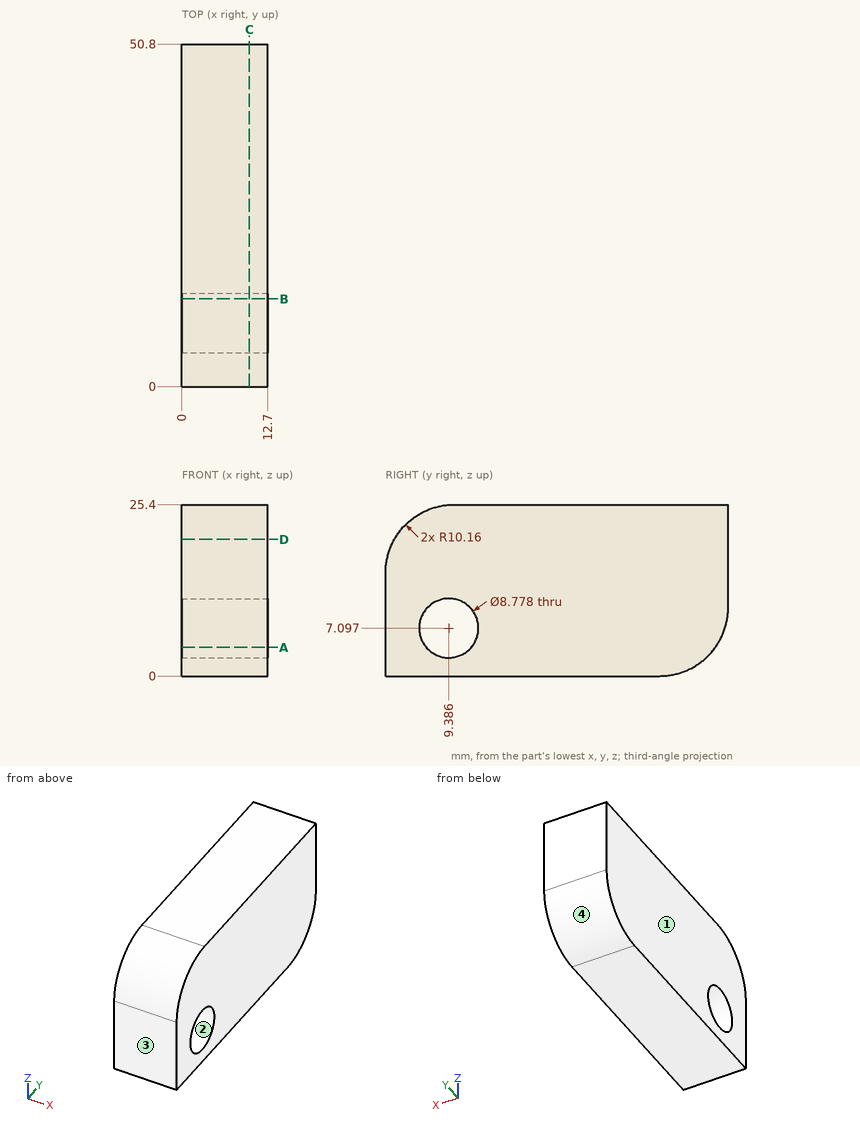
The drawing under review shows one solid part. Ordinate dimensions are in mm from its lowest x, y, z. Coordinates: 2 decimals unless noted, no trailing zeros. Order: outer loops, then holes, each group sorted by start corner. A loop starts at its lowest first (then second) coordinate and runs counter-clockwise, first axis right, second up. Notation, with made-up numbers: (61, -13) -> (81, -13) arc R20 cw to (81, -5) -> close; hole circle Ø7 at (52.25, 50). An arc over 180 degrees is marked (long way). Return JSON: item names as keys, results as strings.
1. For line 1 (Y direction, x = 7.25, z = 3.5); line 2 (Z direction, x = 1.25, y = 11) (1 decimal); line 3 (Y direction, x = 9.5, z = 8), list the stretches that pass through material, from the lowest coordinate up. Write a range as from..to.
Answer block:
{"line 1": "0..6.87, 11.9..48.31", "line 2": "0..3, 11.2..25.4", "line 3": "0..5.09, 13.68..50.57"}
2. We need section D-D on z = 20.25. Write out the cut boundary in (x, y).
Answer block:
{"outline": "(0, 1.32) -> (12.7, 1.32) -> (12.7, 50.8) -> (0, 50.8) -> close"}
3. We need section B-B on y = 13. Write out the cut boundary in (x, z), and give its area (3 significant figures).
Answer block:
{"outline": "(0, 0) -> (12.7, 0) -> (12.7, 4.61) -> (0, 4.61) -> close; (0, 9.59) -> (12.7, 9.59) -> (12.7, 25.4) -> (0, 25.4) -> close", "area": "259 mm²"}
4. The part is to be moulded in two halves that separate along Y. For the marked faces 1, 2, 3 and 4, say which applies: +Y half, -Y half, draft (parallel to the pull), parting line (faces both ways), or undercut.
Answer block:
{"face 1": "draft", "face 2": "undercut", "face 3": "-Y half", "face 4": "+Y half"}
5. For pin 1 Ø4 at (x, z) = (1.5, 21.5) entering from -Y, flat-tipped, find the tip position at first contact; note if it passes through.
Answer block:
{"pin 1": "y = 0.94"}
6. We need section C-C on x = 10. Write out the cut boundary in (y, z) (1 decimal), and give its area (3 significant figures).
Answer block:
{"outline": "(0, 0) -> (40.6, 0) arc R10.2 ccw to (50.8, 10.2) -> (50.8, 25.4) -> (10.2, 25.4) arc R10.2 ccw to (0, 15.2) -> close; hole circle Ø8.8 at (9.4, 7.1)", "area": "1,190 mm²"}
7. We need section A-A on z = 4.25. Write out the cut boundary in (x, y), and give its area (3 significant figures).
Answer block:
{"outline": "(0, 0) -> (12.7, 0) -> (12.7, 6.05) -> (0, 6.05) -> close; (0, 12.73) -> (12.7, 12.73) -> (12.7, 48.9) -> (0, 48.9) -> close", "area": "536 mm²"}
